Input: dimensioned drawing with shaded views. Units: mm. Origin: part minimum x, y, z. A direction names the side the tool comes from. Coordinates: 2 decimals unless noted, no trailing zeros. Order: outer loops, then holes, each group sorted by start corner. A loop starts at its lowest first (then second) coordinate and runs counter-clockwise, first axis right, second up.
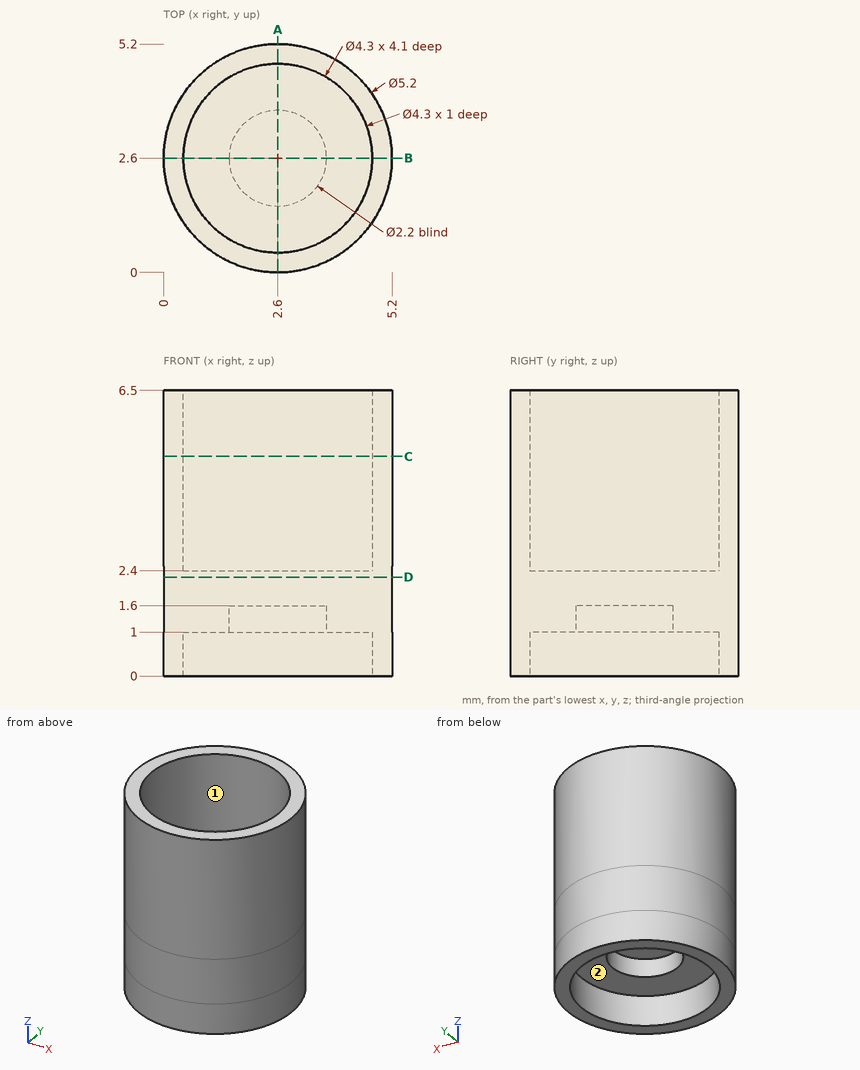
1. Section query A-A, the plane x = 2.6. Output: boundary loops of the cut face in (y, z).
2. Access query for the marked faces 1 and 2. Directions: +Z, -Z, +X, -X, +Y, -Y. A direction counts if a zero-diameter tool reaches every point of the face in a straight line with its end or side. Return the directions, or none.
3. Material intervals for line 1 along Y through (x, z) = (2.6, 4.25); line 2 along X through (y, z) = (2.65, 1.5), sorted ascending.
4. Section query C-C, the plane z = 5. Output: boundary loops of the cut face in (x, y).
5. Contact query for flat-ended pins moving along their axis: P1, Ø1.3, axis at x = 2.6, y = 2.6, coming from the +Z side; P2, Ø1, axis at y = 1.5, z = 4, coming from the +X side; P3, Ø1.8, axis at x = 3, y = 2.5, coming from the -Z side. Output: stop coordinate, or through.
6. Section query D-D, the plane z = 2.25. Output: boundary loops of the cut face in (x, y), plus the area to 3 significant figures.
Answer key:
1. outline: (0, 0) - (0.45, 0) - (0.45, 1) - (1.5, 1) - (1.5, 1.6) - (3.7, 1.6) - (3.7, 1) - (4.75, 1) - (4.75, 0) - (5.2, 0) - (5.2, 6.5) - (4.75, 6.5) - (4.75, 2.4) - (0.45, 2.4) - (0.45, 6.5) - (0, 6.5) - close
2. face 1: +Z
2. face 2: -Z
3. line 1: y = 0 to 0.45, 4.75 to 5.2
3. line 2: x = 0 to 1.5, 3.7 to 5.2
4. outline: circle Ø5.2 at (2.6, 2.6); hole circle Ø4.3 at (2.6, 2.6)
5. P1: stops at z = 2.4
5. P2: stops at x = 5.13
5. P3: stops at z = 1
6. outline: circle Ø5.2 at (2.6, 2.6)
6. area: 21.2 mm2
